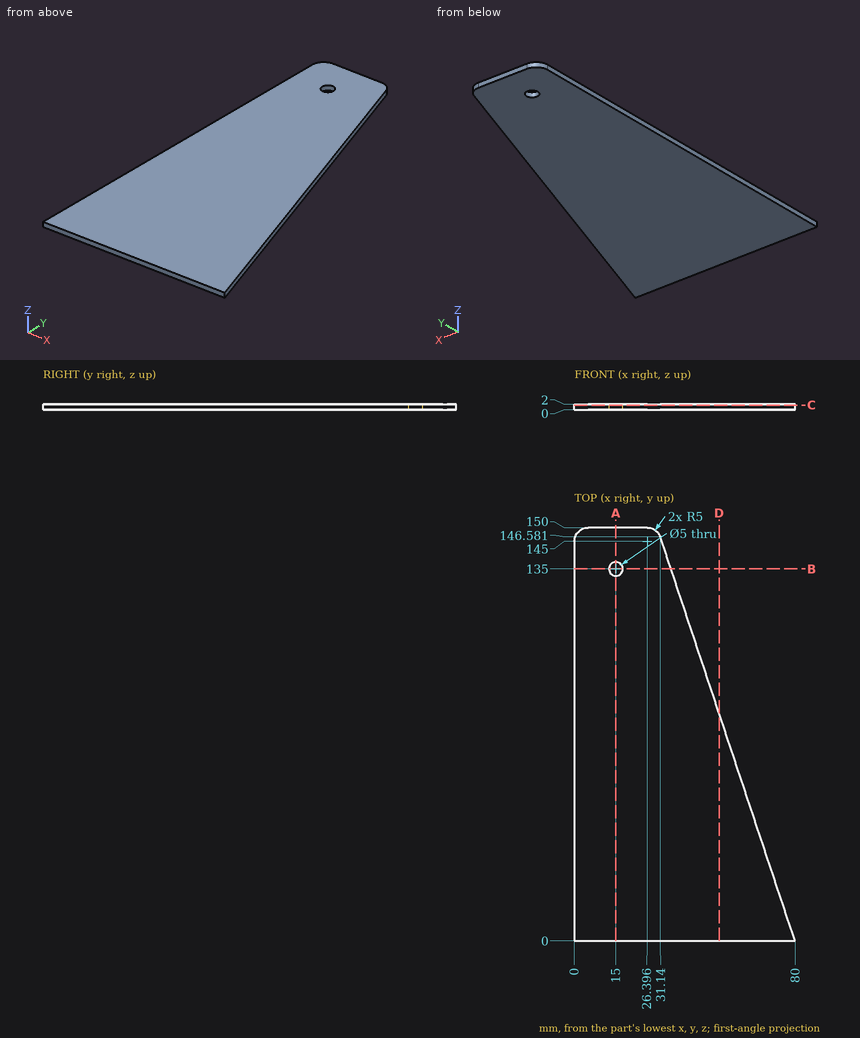
Here's the drawing with two shaded views (mm, measured from the low corner). I have some questions. Give positions to 0.01 mm unless a question says otherwise; leave off trailing zeros. Order: outer loops, then holes, each group sorted by start corner. A loop starts at its lowest first (then second) coordinate and runs counter-clockwise, first axis right, second up. Notation, with made-up numbers: M 26,-34.75 L 83,-34.75 A19 cw 83,-3.75 Z; hole C -34,5 d7. An arc over 180 degrees is marked long. Answer as a JSON object with one key per item and string values. Group by question number.
1) I'm going to push flat-ended pins straight in: pin 1 Ø6 at (x, y) = (10.5, 53) entering from -Z; pin 2 Ø3 at (x, y) = (15, 135) entering from -Z. Where does each tip first touch, or does it pass through?
2) Suppose I cut it at B-B, the plane y = 135. Write out the boundary of the cut face in (x, z).
3) Suppose I cut it at C-C, the plane z = 1.55. Write out the boundary of the cut face in (x, y).
4) Suppose I cut it at A-A, the plane x = 15. Write out the boundary of the cut face in (y, z), plus the area to 3 significant figures.
5) Suppose I cut it at D-D, the plane x = 52.5. Write out the boundary of the cut face in (y, z).
6) Please list where these lines run through material, in increasing order: L1, parallel to Y at x = 15, z = 1.15; L2, parallel to X at y = 135, z = 1.4; L3, parallel to X at y = 85.5, z = 1.75. Write a range as [from, to].
Results found:
{
 "1": {"pin 1": "z = 0", "pin 2": "through"},
 "2": {"outline": "M 0,0 L 12.5,0 L 12.5,2 L 0,2 Z; M 17.5,0 L 35,0 L 35,2 L 17.5,2 Z"},
 "3": {"outline": "M 0,0 L 80,0 L 31.14,146.58 A5 ccw 26.4,150 L 5,150 A5 ccw 0,145 Z; hole C 15,135 d5"},
 "4": {"outline": "M 0,0 L 132.5,0 L 132.5,2 L 0,2 Z; M 137.5,0 L 150,0 L 150,2 L 137.5,2 Z", "area": "290 mm²"},
 "5": {"outline": "M 0,0 L 82.5,0 L 82.5,2 L 0,2 Z"},
 "6": {"L1": "[0, 132.5], [137.5, 150]", "L2": "[0, 12.5], [17.5, 35]", "L3": "[0, 51.5]"}
}
